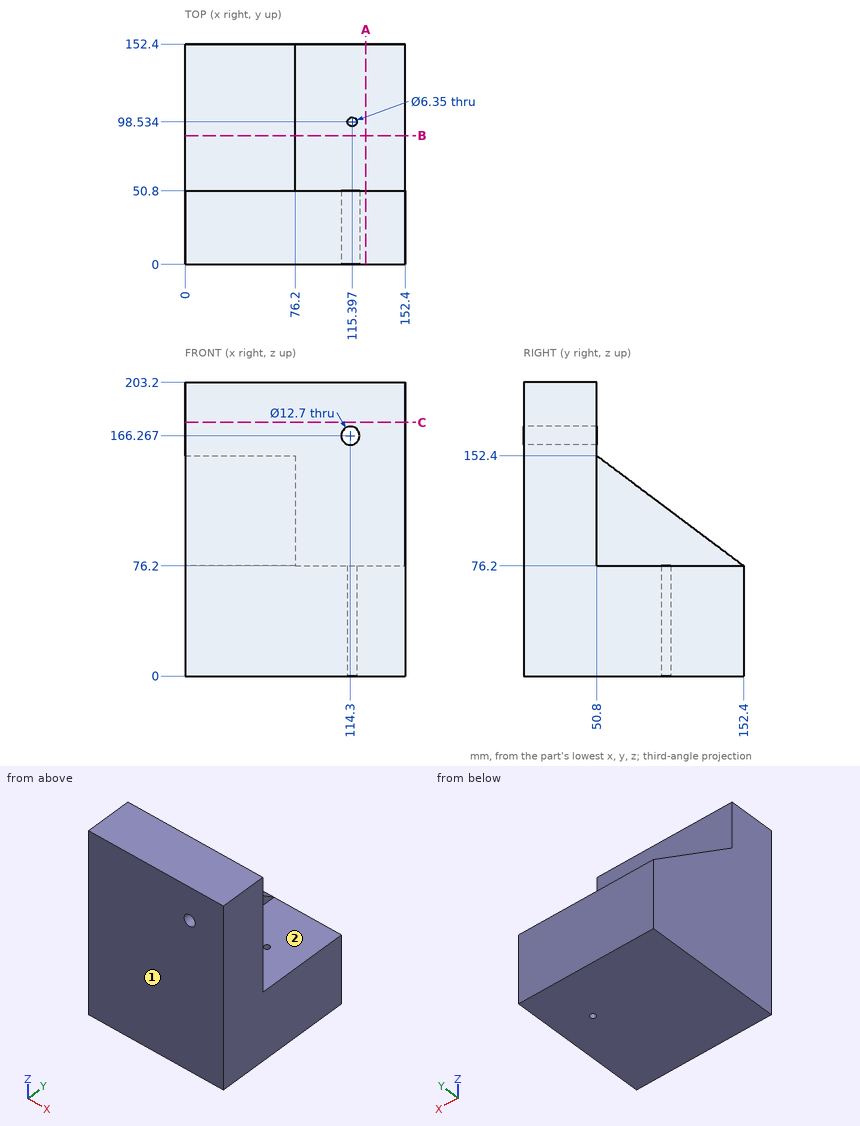
The drawing under review shows one solid part. Ordinate dimensions are in mm from its lowest x, y, z. A direction names the side the tool comes from. Coordinates: 2 decimals unless noted, no trailing zeros. Order: outer loops, then holes, each group sorted by start corner. A loop starts at its lowest first (then second) coordinate and runs counter-clockwise, first axis right, second up. Notation, with made-up numbers: (57.5, 28.5) - (67.5, 28.5) arc R23 cw to (67.5, 62.5) - close; hole circle Ø4 at (51.25, 63). An arc over 180 degrees is marked (long way). Put each result on its own line as item: value.
1) Tool access review of the marked faces 1 and 2: name each direction out of +Z, -Z, +X, -X, +Y, -Y from which nothing blocks a thin tool from reaching the whole face with its end or side.
Response values:
face 1: +Z, -Z, +X, -X, -Y
face 2: +Z, +X, +Y
2) Take a section at A-A, the plane x = 125. Give the boundary of the cut face in (y, z), and give its area (3 significant figures).
Response values:
outline: (0, 0) - (152.4, 0) - (152.4, 76.2) - (50.8, 76.2) - (50.8, 203.2) - (0, 203.2) - close
area: 18,100 mm²
3) Insertion check: P1, Ø1.5, axis at x = 94.5, y = 94.5, coming from the +Z side; P2, Ø10, axis at x = 54.5, z = 136.5, coming from the +Y side; P3, Ø3, axis at x = 60, z = 181, coming from the +Y side. Each pin has a flat end and moves straight along its axis. Give the tip position at first contact, or say it passes through.
Response values:
P1: stops at z = 76.2
P2: stops at y = 78.67
P3: stops at y = 50.8
4) Take a section at C-C, the plane z = 175.5. Give the boundary of the cut face in (x, y).
Response values:
outline: (0, 0) - (152.4, 0) - (152.4, 50.8) - (0, 50.8) - close
5) Take a section at B-B, the plane y = 89. Give the boundary of the cut face in (x, z).
Response values:
outline: (0, 0) - (152.4, 0) - (152.4, 76.2) - (76.2, 76.2) - (76.2, 123.75) - (0, 123.75) - close
6) Wall thickness on L1, parallel to Z at x = 114.3, y = 31; L2, parallel to Y at x = 107.5, z = 191; L3, parallel to Z at x = 119.5, y = 101.5: over which ranges is each line inside the solid? List them lowest first. Write a range as from..to.
Response values:
L1: z = 0..159.92, 172.62..203.2
L2: y = 0..50.8
L3: z = 0..76.2
